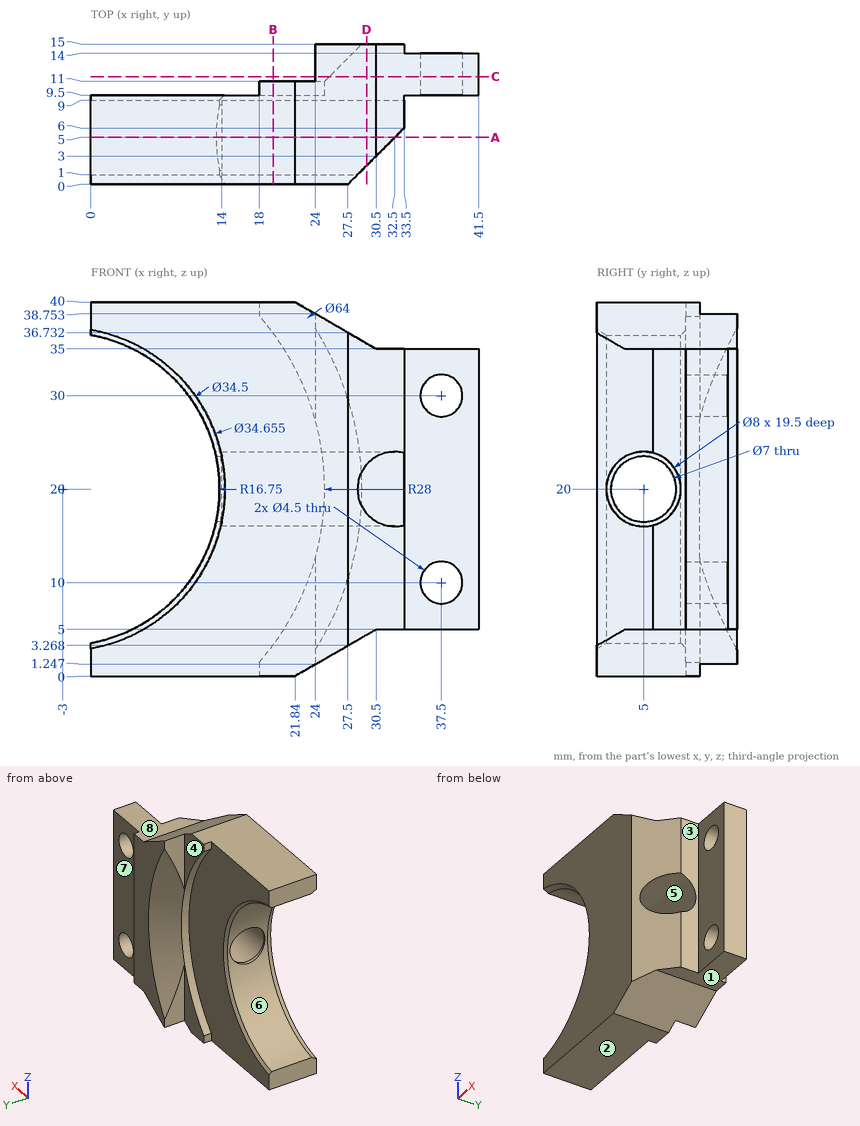
Could you check a few things on this drawing? It's one solid part, dimensions in mm from its lowest x, y, z. A direction names the side the tool comes from. Give positions to 0.01 mm unless a question says otherwise; leave off trailing zeros. Order: outer loops, then holes, each group sorted by start corner. A loop starts at its lowest first (then second) coordinate and runs counter-clockwise, first axis right, second up. Notation, with made-up numbers: (-35, -12.75) - (-6, -12.75) arc R12 ccw to (-6, 7.25) - close; hole circle Ø6 at (42, 50). An arc over 180 degrees is marked (long way). One line per question, with ' | ' between items. Start each with the question number.
Item 1: For the marked faces 1, 2, 3, 4 and 5, which set-ups out of +Z, -Z, +X, -X, +Y, -Y let a thin tool reach every point of the face, with its end or its side?
Item 2: I want a section at B-B on x = 19.5. Write out the boundary of the cut face in (y, z), then the cut area to 3 significant figures.
Item 3: I'm going to push flat-ended pins straight in: pin 1 Ø4.5 at (y, z) = (12.5, 34.5) entering from -X (1 decimal); pin 2 Ø5.5 at (x, y) = (35.5, 11.5) entering from +Z; pin 3 Ø9 at (x, z) = (39.5, 13.5) entering from -Y; pin 4 Ø2 at (x, z) = (8, 7) entering from -Y. Where does each tip first touch, or does it pass through?
Item 4: Thinking about a two-plate mould opening in Z: for the marked faces 6, 7 and 8, which applies, pulls with the +Z half, pulls with the -Z half, needs draft (parallel to the pull), parting line crosses it, or undercut?
Item 5: I want a section at A-A on y = 5. Write out the boundary of the cut face in (x, z), then the cut area to 3 significant figures.
Item 6: I want a section at D-D on x = 29.5. Write out the boundary of the cut face in (y, z).
Item 7: I want a section at C-C on y = 11.5. Write out the boundary of the cut face in (x, z), then the cut area to 3 significant figures.
Item 8: I need wall thicknesses on probe 1 along X at (y, z) = (11.6, 10); probe 2 along Y at (x, z) = (10.5, 31); probe 3 along Y at (x, z) = (24, 20). Which ranges of each line are inside material? Lowest first, please. Write a range as [from, to].
Verdict:
1) face 1: -Z, +X, +Y, -Y | face 2: -Z, +X, -X, +Y, -Y | face 3: +Z, -Z, +X, -Y | face 4: +Z, -Z, -X, +Y | face 5: +X
2) outline: (0, 0) - (11, 0) - (11, 3.33) - (9.5, 3.33) - (9.5, 36.67) - (11, 36.67) - (11, 40) - (0, 40) - close; hole circle Ø8 at (5, 20) | area: 340 mm^2
3) pin 1: x = 19.9 | pin 2: z = 35 | pin 3: y = 9.5 | pin 4: y = 0
4) face 6: undercut | face 7: needs draft | face 8: pulls with the +Z half
5) outline: (0, 0) - (21.84, 0) - (30.5, 5) - (32.5, 5) - (32.5, 16) - (14, 16) - (14, 16.5) - (13.38, 16.5) arc R16.75 cw to (0, 3.52) - close; (0, 36.48) arc R16.75 cw to (13.38, 23.5) - (14, 23.5) - (14, 24) - (32.5, 24) - (32.5, 35) - (30.5, 35) - (21.84, 40) - (0, 40) - close | area: 745 mm^2
6) outline: (2, 4.42) - (15, 4.42) - (15, 35.58) - (2, 35.58) - (2, 22.65) arc R4 cw (long way) to (2, 17.35) - close
7) outline: (24, 1.25) - (30.5, 5) - (41.5, 5) - (41.5, 35) - (30.5, 35) - (24, 38.75) - (24, 29.12) arc R28.5 cw to (24, 10.88) - close; hole circle Ø4.5 at (37.5, 10); hole circle Ø4.5 at (37.5, 30) | area: 499 mm^2
8) probe 1: [24, 35.25], [39.75, 41.5] | probe 2: [0, 9.5] | probe 3: [0, 1], [9, 9.5]
